Autodesk Inventor part; units mm, degrees
ref_plane "YZ Plane" through (0, 0, 0) normal (1, 0, 0) x (0, 1, 0)
ref_plane "XZ Plane" through (0, 0, 0) normal (0, 1, 0) x (-1, 0, 0)
ref_plane "XY Plane" through (0, 0, 0) normal (0, 0, 1) x (1, 0, 0)
sketch "Sketch1" plane through (0, 0, 0) normal (0, 1, 0) x (-1, 0, 0)
  line L0 (0, 0) -> (-20, 0)
  line L1 (-20, 0) -> (-20, -20)
  line L2 (-20, -20) -> (0, -20)
  line L3 (0, -20) -> (0, 0)
  dimension "d0" = 20
  dimension "d1" = 20
extrude "Extrusion1" add sketch "Sketch1" along normal blind 4
sketch "Sketch2" plane through (0, 4, 0) normal (0, 1, 0) x (1, 0, 0)
  line L0 (0, 0) -> (20, 0)
  line L1 (20, 0) -> (20, 4)
  line L2 (20, 4) -> (4, 4)
  line L3 (0, 4) -> (0, 0)
  line L4 (0, 0) -> (4, 0)
  line L5 (4, 20) -> (0, 20)
  line L6 (0, 20) -> (0, 0)
  line L7 (4, 4) -> (4, 20)
  line L8 (0, 0) -> (20, 0)
  line L9 (0, 0) -> (20, 0)
  line L10 (0, 20) -> (0, 0)
  line L11 (0, 0) -> (0, 20)
extrude "Extrusion2" add sketch "Sketch2" along normal blind 45
hole "Hole2" at (12, 12, -4) direction (0, 0, 1) diameter 4 end through all
hole "Hole3" at (4, 12, -12) direction (-1, 0, 0) diameter 4 end through all
hole "Hole4" at (12, 4, -12) direction (0, -1, 0) diameter 4 end through all
sketch "Sketch3" plane through (20, 4, -4) normal (0, 0, -1) x (-1, 0, 0)
  line L0 (12.0415, 8) -> (10.0207, 4.5)
  line L1 (10.0207, 4.5) -> (5.9793, 4.5)
  line L2 (5.9793, 4.5) -> (3.9585, 8)
  line L3 (3.9585, 8) -> (5.9793, 11.5)
  line L4 (5.9793, 11.5) -> (10.0207, 11.5)
  line L5 (10.0207, 11.5) -> (12.0415, 8)
  point P0 (20, -4)
  point P1 (8, 8)
  dimension "d51" = 7
sketch "Sketch4" plane through (4, 4, -4) normal (1, 0, 0) x (0, 0, -1)
  line L0 (12.0415, 8) -> (10.0207, 4.5)
  line L1 (10.0207, 4.5) -> (5.9793, 4.5)
  line L2 (5.9793, 4.5) -> (3.9585, 8)
  line L3 (3.9585, 8) -> (5.9793, 11.5)
  line L4 (5.9793, 11.5) -> (10.0207, 11.5)
  line L5 (10.0207, 11.5) -> (12.0415, 8)
  point P0 (-4, -4)
  point P1 (8, 8)
  dimension "d52" = 7
sketch "Sketch5" plane through (0, 4, 0) normal (0, 1, 0) x (1, 0, 0)
  circle A0 centre (12, 12) radius 2
  line L0 (12, 7.9585) -> (8.5, 9.9793)
  line L1 (8.5, 9.9793) -> (8.5, 14.0207)
  line L2 (8.5, 14.0207) -> (12, 16.0415)
  line L3 (12, 16.0415) -> (15.5, 14.0207)
  line L4 (15.5, 14.0207) -> (15.5, 9.9793)
  line L5 (15.5, 9.9793) -> (12, 7.9585)
  point P0 (0, 0)
  dimension "d53" = 7
extrude "Extrusion3" cut sketch "Sketch3" against normal blind 3.2
extrude "Extrusion4" cut sketch "Sketch4" against normal blind 3.2
extrude "Extrusion5" cut sketch "Sketch5" against normal blind 3.2
sketch "Sketch6" plane through (0, 49, 0) normal (0, 1, 0) x (1, 0, 0)
  line L0 (0, 0) -> (20, 0)
  line L1 (0, 0) -> (0, 46)
  line L2 (0, 20) -> (0, 0)
  line L3 (0, 0) -> (46, 0)
  line L4 (46, 0) -> (46, 14)
  line L5 (0, 46) -> (14, 46)
  line L6 (14, 46) -> (14, 14)
  line L7 (14, 14) -> (46, 14)
  line L8 (20, 4) -> (4, 4)
  line L9 (4, 4) -> (4, 20)
  line L10 (20, 20) -> (4, 20)
  line L11 (20, 4) -> (20, 20)
  point P0 (9.5, 9.5)
  point P1 (9.5, 40.5)
  point P2 (40.5, 9.5)
  dimension "d62" = 14
  dimension "d65" = 42
  dimension "d66" = 42
  dimension "d68" = 5.5
  dimension "d69" = 5.5
  dimension "d70" = 31
  dimension "d71" = 31
  dimension "d72" = 14
extrude "Extrusion6" add sketch "Sketch6" along normal blind 6 contours L1 L5 L6 L10 L9 L8 L11 L7 L4 L3 L0 | L11 L8 L9 L10 L6 L7
hole "Hole5" at (9.5, 49, -9.5) at (9.5, 49, -40.5) at (40.5, 49, -9.5) direction (0, 1, 0) diameter 3 end through all
sketch "Sketch7" plane through (0, 55, 0) normal (0, 1, 0) x (1, 0, 0)
  line L0 (0, 0) -> (20, 0)
  line L1 (20, 4) -> (4, 4)
  line L2 (0, 0) -> (20, 0)
  line L3 (20, 0) -> (20, 4)
  line L4 (20, 4) -> (4, 4)
  line L5 (0, 4) -> (0, 0)
  line L6 (0, 0) -> (4, 0)
  line L7 (4, 20) -> (0, 20)
  line L8 (0, 20) -> (0, 0)
  line L9 (4, 4) -> (4, 20)
  dimension "d82" = 20
  dimension "d83" = 4
  dimension "d84" = 4
  dimension "d85" = 20
extrude "Extrusion7" add sketch "Sketch7" along normal blind 16
hole "Hole6" at (12, 63, -4) direction (0, 0, 1) diameter 4 end through all
hole "Hole7" at (4, 63, -12) direction (-1, 0, 0) diameter 4 end through all
sketch "Sketch8" plane through (4, 55, -4) normal (1, 0, 0) x (0, 0, -1)
  line L0 (3.9585, 8) -> (5.9793, 11.5)
  line L1 (5.9793, 11.5) -> (10.0207, 11.5)
  line L2 (10.0207, 11.5) -> (12.0415, 8)
  line L3 (12.0415, 8) -> (10.0207, 4.5)
  line L4 (10.0207, 4.5) -> (5.9793, 4.5)
  line L5 (5.9793, 4.5) -> (3.9585, 8)
  point P0 (-4, -55)
  point P1 (8, 8)
  dimension "d106" = 7
sketch "Sketch9" plane through (20, 55, -4) normal (0, 0, -1) x (-1, 0, 0)
  circle A0 centre (8, 8) radius 2
  line L0 (3.9585, 8) -> (5.9793, 11.5)
  line L1 (5.9793, 11.5) -> (10.0207, 11.5)
  line L2 (10.0207, 11.5) -> (12.0415, 8)
  line L3 (12.0415, 8) -> (10.0207, 4.5)
  line L4 (10.0207, 4.5) -> (5.9793, 4.5)
  line L5 (5.9793, 4.5) -> (3.9585, 8)
  point P0 (20, -55)
  dimension "d107" = 7
extrude "Extrusion8" cut sketch "Sketch9" against normal blind 3.2
extrude "Extrusion9" cut sketch "Sketch8" against normal blind 3.2
hole "Hole8" at (25, 55, -7) direction (0, -1, 0) diameter 8 end through all
properties part number "MotorMountRight" material "PLA Orange"
Work out the finished part from the listing and answer in its coordinate system (mm). A direction names the side the tool comes from. Round coordinates to 2 decimals unless told otherwise and drop trailing zeros. Write each loop counter-clockwise with the first axis right and the second up, starting at its lowest first coordinate (ties: lowest second). Pieces come first, ordered by that corner, then holes. Notation, with made-up numbers: (7.25, 5.5) - (20.25, 5.5) arc R16 cw to (20.25, 28.5) - close; hole circle Ø2 at (-23, -9.5). An arc over 180 degrees is marked (long way). Answer in a Markdown table with one row per item. Add a question column.
1. A cutting plane is placed at A-A, the plane x = 40.5. Determine the outline of the cut face in (y, z).
2. A cutting plane is placed at D-D, the plane z = -40.5. Determine the outline of the cut face in (x, y), and give its area (3 significant figures).
3. A cutting plane is placed at C-C, the plane x = 3. Determine the outline of the cut face in (y, z), and give its area (3 significant figures).
4. For faces 1 (the flat face through (13.726, 2.422, -15.045)), 2 (the flat face through (0.8, 65, -14)), 3 (the flat face through (12, 59.5, -2)), 4 (the flat face through (12, 59, -4)), determine the directions among +Z, -Z, +X, -X, +Y, -Y from which every point of the face is accessible in a straight line to the end or side of a thin tool.
5. A cutting plane is placed at B-B, the plane z = -12. Count the separate pieces of the cut face and the enclosed holes in it, and give its area (3 significant figures).
6. Given pin 1 (13 mm diameter, centred on x = 12, y = 64.5, fed in from -Z); pin 2 (6 mm diameter, centred on y = 14, z = -5, fed in from +X); pin 3 (1.5 mm diameter, centred on y = 34, z = -14.5, fed in from +X); pin 4 (10 mm diameter, centred on x = 27, y = 60.5, fed in from +Z), each flat-ended and moving along its own axis, determine where each tip first touches the part or whether it passes through.
7. The mould has two halves that part along Y. Classify faces 5 (the cylindrical face through (10.648, 0.394, -13.474)), 6 (the flat face through (2, 8.5, -12)): +Y half, -Y half, draft (parallel to the pull), parting line (faces both ways), or undercut.
8. Find the intervals of material crossed by line 1 along Y through (x, z) = (0.3, -12); line 2 along X through (y, z) = (50.8, -7); line 3 along X through (y, z) = (50, -9), in increasing order. Write a range as from..to.
Worked out:
| question | item | result |
|---|---|---|
| 1 | outline | (49, -14) - (55, -14) - (55, -11) - (49, -11) - close; (49, -8) - (55, -8) - (55, 0) - (49, 0) - close |
| 2 | outline | (0, 49) - (8, 49) - (8, 55) - (0, 55) - close; (11, 49) - (14, 49) - (14, 55) - (11, 55) - close |
| 2 | area | 66.0 mm^2 |
| 3 | outline | (0, -20) - (49, -20) - (49, -46) - (55, -46) - (55, -20) - (71, -20) - (71, 0) - (0, 0) - close; hole (8.5, -14.02) - (12, -16.04) - (15.5, -14.02) - (15.5, -9.98) - (12, -7.96) - (8.5, -9.98) - close; hole (59.5, -14.02) - (63, -16.04) - (66.5, -14.02) - (66.5, -9.98) - (63, -7.96) - (59.5, -9.98) - close |
| 3 | area | 1,490 mm^2 |
| 4 | face 1 | none |
| 4 | face 2 | +X |
| 4 | face 3 | -Z |
| 4 | face 4 | -Z, +X, +Y |
| 5 | separate pieces | 4 |
| 5 | enclosed holes | 0 |
| 5 | area | 523 mm^2 |
| 6 | pin 1 | z = -4 |
| 6 | pin 2 | x = 20 |
| 6 | pin 3 | x = 4 |
| 6 | pin 4 | through |
| 7 | face 5 | draft |
| 7 | face 6 | undercut |
| 8 | line 1 | 0..10, 14..61, 65..71 |
| 8 | line 2 | 0..21, 29..46 |
| 8 | line 3 | 0..8.09, 10.91..21.54, 28.46..39.09, 41.91..46 |
